```python
from build123d import *

# Parameters (mm, degrees)
SKETCH1_W           = 43
SKETCH1_H           = 43
BOSS_EXTRUDE1_DEPTH = 45
SKETCH3_R           = 3
SKETCH3_R_2         = 7.25
CUT_EXTRUDE4_DEPTH  = 38
SKETCH6_W           = 39
SKETCH6_H           = 39
CUT_EXTRUDE5_DEPTH  = 22
SKETCH7_W           = 43
SKETCH7_H           = 43
SKETCH7_W_2         = 18.4
SKETCH7_H_2         = 18.4
CUT_EXTRUDE8_DEPTH  = 12
FILLET2_R           = 5
FILLET3_R           = 3
SKETCH10_W          = 20.235048465
SKETCH10_H          = 19.323901817
CUT_EXTRUDE9_DEPTH  = 7


with BuildPart() as part:
    # Sketch1 → Boss-Extrude1 (new body)
    with BuildSketch(Plane(origin=(0, 0, 0), x_dir=(0, 1, 0), z_dir=(0, 0, 1))):
        with Locations((-19.5, 19.5)):
            Rectangle(SKETCH1_W, SKETCH1_H)
    extrude(amount=BOSS_EXTRUDE1_DEPTH)

    # Sketch3 → Cut-Extrude4 (cut)
    with BuildSketch(Plane.XY.offset(45)):
        with Locations((-20, -3.506761261)):
            Circle(SKETCH3_R)
        with Locations((-20, -19)):
            Circle(SKETCH3_R_2)
        with BuildLine():
            Line((-6, -13), (-6, -25))
            ThreePointArc((-6, -25), (-3, -28), (0, -25))
            Line((0, -25), (0, -13))
            ThreePointArc((0, -13), (-3, -10), (-6, -13))
        make_face()
        with BuildLine():
            Line((-33, -13), (-33, -25))
            ThreePointArc((-33, -25), (-36, -28), (-39, -25))
            Line((-39, -25), (-39, -13))
            ThreePointArc((-39, -13), (-36, -10), (-33, -13))
        make_face()
    extrude(amount=-CUT_EXTRUDE4_DEPTH, mode=Mode.SUBTRACT)

    # Sketch6 → Cut-Extrude5 (cut)
    with BuildSketch(Plane.XY.offset(45)):
        with Locations((-19.5, -19.5)):
            Rectangle(SKETCH6_W, SKETCH6_H)
    extrude(amount=-CUT_EXTRUDE5_DEPTH, mode=Mode.SUBTRACT)

    # Sketch7 → Cut-Extrude8 (cut)
    with BuildSketch(Plane(origin=(0, 0, 0), x_dir=(1, 0, 0), z_dir=(0, 0, -1))):
        with Locations((-19.5, 19.5)):
            Rectangle(SKETCH7_W, SKETCH7_H)
        with Locations((-20.012556467, 19.015852406)):
            Rectangle(SKETCH7_W_2, SKETCH7_H_2, mode=Mode.SUBTRACT)
    extrude(amount=-CUT_EXTRUDE8_DEPTH, mode=Mode.SUBTRACT)

    # Fillet2
    fillet2_edges = [part.edges().sort_by_distance(p)[0] for p in [
        (-10.812556467, -9.815852406, 6),
        (-10.812556467, -28.215852406, 6),
        (-29.212556467, -28.215852406, 6),
        (-29.212556467, -9.815852406, 6),
    ]]
    fillet(fillet2_edges, radius=FILLET2_R)

    # Fillet3
    fillet3_edges = [part.edges().sort_by_distance(p)[0] for p in [
        (-41, -41, 28.5),
        (2, -41, 28.5),
        (2, 2, 28.5),
        (-41, 2, 28.5),
    ]]
    fillet(fillet3_edges, radius=FILLET3_R)

    # Sketch10 → Cut-Extrude9 (cut)
    with BuildSketch(Plane(origin=(0, 0, 0), x_dir=(1, 0, 0), z_dir=(0, 0, -1))):
        with Locations((-19.898626658, 18.797657793)):
            Rectangle(SKETCH10_W, SKETCH10_H)
    extrude(amount=-CUT_EXTRUDE9_DEPTH, mode=Mode.SUBTRACT)


solid = part.part
```
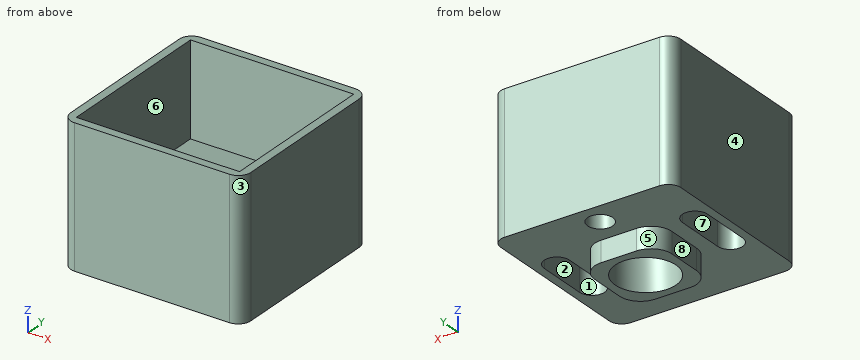
CAD build for the part. Positions are in the model's coordinates, mm. Face numbers are marked on the shaded views. A direction names the side the tool comes from. Round coordinates to 2 decimals unless told otherwise and drop trailing zeros. Loops run counter-clockwise (first coordinate to the right, second up) from the corner with the lowest first, then second, coordinate; pieces in that order, holes last. Notation, with made-up numbers: M 50,29 L 71,29 A15 ccw 71,35 Z; hole C 26.25,-8.75 d1. An arc over 180 degrees is marked long. Return JSON: item names as keys, results as strings. Group by question number.
(1) Drop flat-ended pins along their axis: P1, Ø8, axis at x = -13.5, y = -21, coming from the +Z side; P2, Ø1.5, axis at y = -17.5, z = 10.5, coming from the +X side; P3, Ø8, axis at x = -20, y = -3.51, coming from the -Z side. Give the stop position or say it passes through.
(2) Saw through at C-C, the plane x = -36. List the corners of the cut face in (y, z).
(3) Saw through at D-D, the plane z = 34. List the corners of the cut face in (x, y), and give its area (3 significant figures).
(4) Saw through at B-B, the plane y = -37. List the corners of the cut face in (x, z).
(5) Tool access for the marked faces 5, 6, 7 and 8: list every direction of +Z, -Z, +X, -X, +Y, -Y with a clear straight run to the whole face (end or side of a thin tool).
(6) Wall check: probe 1 along Y at (x, z) = (-20, 14.5); probe 2 along X at (y, z) = (-36.5, 43). Give the ranges that are in metal, low to high. Write a range as [from, to].
(7) Saw through at A-A, the plane x = -20. List the corners of the cut face in (y, z), and give its area (3 significant figures).
(8) Mould opens along Y. For the marked faces 1, 2, 3 and 4 say: +Y half, -Y half, draft (parallel to the pull), parting line (faces both ways), or undercut.
Answer list:
{
 "1": {"P1": "z = 23", "P2": "x = -10.81", "P3": "z = 12"},
 "2": {"outline": "M -41,12 L -28,12 L -28,23 L -39,23 L -39,45 L -41,45 Z; M -10,12 L 2,12 L 2,45 L 0,45 L 0,23 L -10,23 Z"},
 "3": {"outline": "M -41,-38 A3 ccw -38,-41 L -1,-41 A3 ccw 2,-38 L 2,-1 A3 ccw -1,2 L -38,2 A3 ccw -41,-1 Z; hole M -39,-39 L 0,-39 L 0,0 L -39,0 Z", "area": "320 mm2"},
 "4": {"outline": "M -41,12 L 2,12 L 2,45 L 0,45 L 0,23 L -39,23 L -39,45 L -41,45 Z"},
 "5": {"face 5": "-Z, -X, +Y", "face 6": "+Z", "face 7": "+Z, -Z", "face 8": "-Z, -X, +Y, -Y"},
 "6": {"probe 1": "[-41, -26.25], [-11.75, -6.51], [-0.51, 2]", "probe 2": "[-41, -39], [0, 2]"},
 "7": {"outline": "M -41,12 L -28.22,12 L -28.22,7 L -26.25,7 L -26.25,23 L -39,23 L -39,45 L -41,45 Z; M -11.75,7 L -9.82,7 L -9.82,12 L -6.51,12 L -6.51,23 L -11.75,23 Z; M -0.51,12 L 2,12 L 2,45 L 0,45 L 0,23 L -0.51,23 Z", "area": "355 mm2"},
 "8": {"face 1": "undercut", "face 2": "undercut", "face 3": "-Y half", "face 4": "draft"}
}
